```python
from build123d import *

# Parameters (mm, degrees)
F0_R      = 40
F1_DEPTH  = 30
F1_FACE_R = 40
F2_DEPTH  = 30
F2_TAPER  = 26
F3_R      = 20.1
F4_DEPTH  = 60.001


with BuildPart() as f1:
    # F0 (on Front) → F1 (new body)
    with BuildSketch(Plane.XZ):
        Circle(F0_R)
    extrude(amount=F1_DEPTH)

    # F1_face (on face) → F2 (join)
    with BuildSketch(Plane.XZ.offset(30)):
        Circle(F1_FACE_R)
    extrude(amount=F2_DEPTH, taper=F2_TAPER)

    # F3 (on face) → F4 (cut, through all)
    with BuildSketch(Plane.XZ.offset(60)):
        Circle(F3_R)
    extrude(amount=-F4_DEPTH, mode=Mode.SUBTRACT)


solid = f1.part
```
Could you check a few things on this model? Use its own coordinates, in mm. Round coordinates to 2 decimals unless told otherwise and drop trailing zeros. Loops run counter-clockwise (first coordinate to the right, second up) from the corner with the lowest first, then second, coordinate; pieces in that order, holes last. Notation, with made-up numbers: (18, 23) - (67, 23) arc R35 cw to (67, 57) - close; hole circle Ø4 at (-23.5, 18.5). An arc over 180 degrees is marked (long way). Answer in a Markdown table with one row per item. Add a question column.
(1) I'm going to push flat-ended pins straight in: pin 1 (1 mm diameter, centred on y = -15.5, z = -24.5, fed in from +X); pin 2 (10 mm diameter, centred on y = -30.5, z = 17.5, fed in from -X); pin 3 (4 mm diameter, centred on x = -20.5, z = -29, fed in from -Y). Where does each tip first touch, or does it pass through?
(2) If we section it at A-A (y = -8): Please give me the cut outline in (x, z), plus the area to 3 significant figures.
(3) I need wall thicknesses on line 1 along Z through (x, y) = (0, -14); line 2 along Z through (x, y) = (17.5, -51); line 3 along Z through (x, y) = (-29, -3). Which ranges of each line are inside material? Lowest first, please.
(4) If we mould it in two halves opening along Z, with no side actions, what happens to faces 1 (the face through (-8.67, -14.79, -39.05)), 2 (the face through (-9.4, 0, 18.3)), 3 (the face through (19.17, -30.42, 6.04))? For each: pulls with the +Z half, pulls with the -Z half, needs draft (parallel to the pull), parting line crosses it, or undercut.
(5) If we section it at B-B (y = -35): Please give me the cut outline in (x, z).
Model answer:
| question | item | result |
|---|---|---|
| 1 | pin 1 | stops at x = 32 |
| 1 | pin 2 | stops at x = -37.99 |
| 1 | pin 3 | stops at y = -43.3 |
| 2 | outline | circle Ø80 at (0, 0); hole circle Ø40.2 at (0, 0) |
| 2 | area | 3,760 mm² |
| 3 | line 1 | z = -40 to -20.1, 20.1 to 40 |
| 3 | line 2 | z = -24.07 to -9.89, 9.89 to 24.07 |
| 3 | line 3 | z = -27.55 to 27.55 |
| 4 | face 1 | parting line crosses it |
| 4 | face 2 | needs draft |
| 4 | face 3 | undercut |
| 5 | outline | circle Ø75.12 at (0, 0); hole circle Ø40.2 at (0, 0) |
